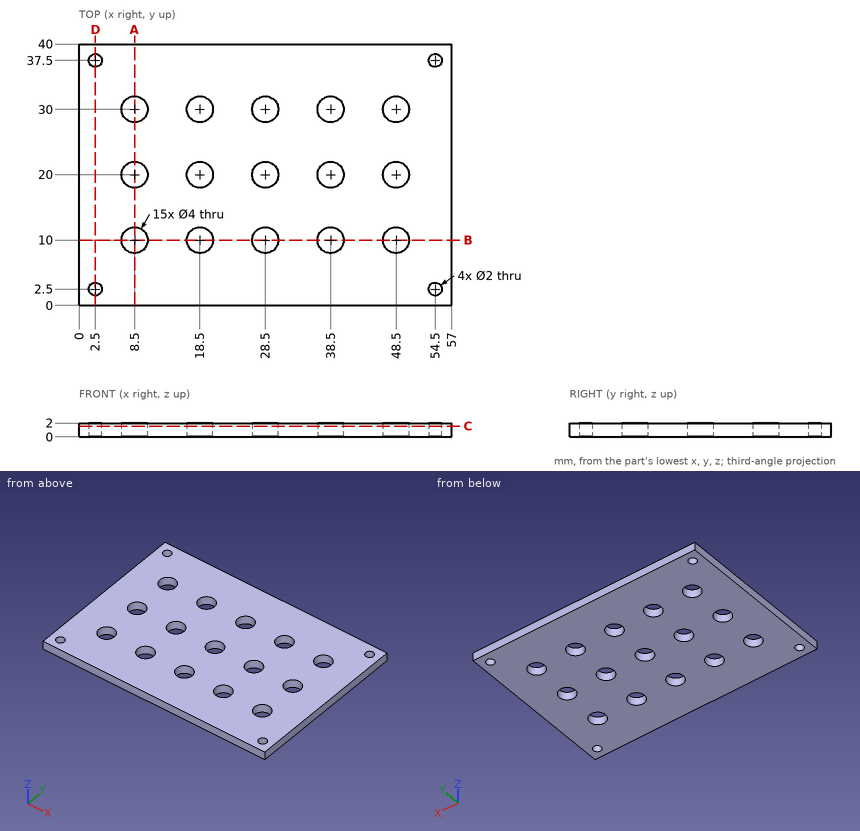
Print and shaded views of the part. All mm, measured from the part's lowest x, y and z. Give positions to 0.01 mm unless a question says otherwise; leave off trailing zeros. Order: outer loops, then holes, each group sorted by start corner. A loop starts at its lowest first (then second) coordinate and runs counter-clockwise, first axis right, second up. Notation, with made-up numbers: (-32.5, 48.5) - (11.5, 48.5) arc R14 ccw to (11.5, 67.5) - close; hole circle Ø4 at (53.25, 62.25). An arc over 180 degrees is marked (long way). Use a Markdown table: item, result.
1) Saw through at C-C on z = 1.6. Count the separate pieces of the cut face and the enclosed holes in it, plus the area to 3 significant figures.
Checked values:
| item | result |
|---|---|
| separate pieces | 1 |
| enclosed holes | 19 |
| area | 2,080 mm² |
2) Saw through at D-D on x = 2.5. List the corners of the cut face in (y, z).
Checked values:
| item | result |
|---|---|
| outline | (0, 0) - (1.5, 0) - (1.5, 2) - (0, 2) - close; (3.5, 0) - (36.5, 0) - (36.5, 2) - (3.5, 2) - close; (38.5, 0) - (40, 0) - (40, 2) - (38.5, 2) - close |
3) Saw through at A-A on x = 8.5. List the corners of the cut face in (y, z).
Checked values:
| item | result |
|---|---|
| outline | (0, 0) - (8, 0) - (8, 2) - (0, 2) - close; (12, 0) - (18, 0) - (18, 2) - (12, 2) - close; (22, 0) - (28, 0) - (28, 2) - (22, 2) - close; (32, 0) - (40, 0) - (40, 2) - (32, 2) - close |
4) Probe L1, parallel to X at y = 20, z = 0.65; L2, parallel to Y at x = 8.5, z = 1.5; L3, parallel to Y at x = 49, z = 1.1. List the from-to ranges inside material, lowest first. Write a range as from..to.
Checked values:
| item | result |
|---|---|
| L1 | 0..6.5, 10.5..16.5, 20.5..26.5, 30.5..36.5, 40.5..46.5, 50.5..57 |
| L2 | 0..8, 12..18, 22..28, 32..40 |
| L3 | 0..8.06, 11.94..18.06, 21.94..28.06, 31.94..40 |
5) Saw through at B-B on y = 10. List the corners of the cut face in (x, z).
Checked values:
| item | result |
|---|---|
| outline | (0, 0) - (6.5, 0) - (6.5, 2) - (0, 2) - close; (10.5, 0) - (16.5, 0) - (16.5, 2) - (10.5, 2) - close; (20.5, 0) - (26.5, 0) - (26.5, 2) - (20.5, 2) - close; (30.5, 0) - (36.5, 0) - (36.5, 2) - (30.5, 2) - close; (40.5, 0) - (46.5, 0) - (46.5, 2) - (40.5, 2) - close; (50.5, 0) - (57, 0) - (57, 2) - (50.5, 2) - close |
